The listing builds one solid part. Answer for the finished solid, in the listing's coordinates (mm). Round coordinates to 2 decimals unless told otherwise and drop trailing zeros. Write each loop counter-clockwise with the first axis right and the second up, starting at its lowest first coordinate (ties: lowest second). Pieces come first, ordered by that corner, then holes.
(1) A cutting plane is placed at C-C, the plane z = 4. Give the vertices of the cut face in (x, y), and give its area (3 significant figures).
(2) A cutting plane is placed at B-B, the plane x = 116. Give the vertices of the cut face in (y, z), and give its area (3 significant figures).
(3) Each of these flat-tipped pins is pushed along its axis until it touches: pin 1 Ø2 at (y, z) = (-31, 8.5) entering from -X; pin 2 Ø4 at (x, y) = (29.5, -17) entering from -Z; pin 3 Ø10 at (x, y) = (32, -11) entering from -Z. Where does it stop, or does it pass through?
(4) A cutting plane is placed at A-A, the plane y = -18.5. Give the vertices of the cut face in (x, z).
(5) Find the intervals of material crossed by probe 1 along Z at (x, y) = (15, -35); probe 2 along Z at (x, y) = (119, -37); probe 3 along X at (y, z) = (-20.5, 7), in increasing order.
from build123d import *

# Parameters (mm, degrees)
SKETCH1_W           = 135.6
SKETCH1_H           = 83.6
BOSS_EXTRUDE1_DEPTH = 57
CUT_EXTRUDE2_DEPTH  = 84.6
FILLET2_R           = 10
FILLET3_R           = 5


with BuildPart() as part:
    # Sketch1 → Boss-Extrude1 (new body)
    with BuildSketch(Plane.XY):
        with Locations((67.8, -41.8)):
            Rectangle(SKETCH1_W, SKETCH1_H)
    extrude(amount=BOSS_EXTRUDE1_DEPTH)

    # Sketch3 → Cut-Extrude2 (cut, through all)
    with BuildSketch(Plane(origin=(0, 0, 0), x_dir=(1, 0, 0), z_dir=(0, 1, 0))):
        Polygon((100.6, 0), (135.6, 0), (135.6, -20.4), align=None)
        Polygon((35, 0), (0, 0), (0, -20.4), align=None)
    extrude(amount=-CUT_EXTRUDE2_DEPTH, mode=Mode.SUBTRACT)

    # Fillet2
    fillet2_edges = [part.edges().sort_by_distance(p)[0] for p in [
        (100.6, -41.8, 0),
        (35, -41.8, 0),
    ]]
    fillet(fillet2_edges, radius=FILLET2_R)

    # Fillet3
    fillet3_edges = [part.edges().sort_by_distance(p)[0] for p in [
        (135.6, -41.8, 20.4),
        (0, -41.8, 20.4),
    ]]
    fillet(fillet3_edges, radius=FILLET3_R)


solid = part.part
Solutions:
1. outline: (28.14, -83.6) - (107.46, -83.6) - (107.46, 0) - (28.14, 0) - close
1. area: 6,630 mm2
2. outline: (-83.6, 8.98) - (0, 8.98) - (0, 57) - (-83.6, 57) - close
2. area: 4,010 mm2
3. pin 1: stops at x = 18.7
3. pin 2: stops at z = 2.04
3. pin 3: stops at z = 0.02
4. outline: (0, 23.27) arc R5 ccw to (2.48, 18.95) - (32.67, 1.36) arc R10 ccw to (37.7, 0) - (97.9, 0) arc R10 ccw to (102.93, 1.36) - (133.12, 18.95) arc R5 ccw to (135.6, 23.27) - (135.6, 57) - (0, 57) - close
5. probe 1: z = 11.66 to 57
5. probe 2: z = 10.72 to 57
5. probe 3: x = 22.99 to 112.61
